The model under review builds one solid part; all positions refer to its coordinate system, in mm. A direction names the side the tool comes from. Give positions to 0.01 mm unless a question says otherwise; leave off trailing zeros. Loops run counter-clockwise (first coordinate to the right, second up) from the corner with the lowest first, then second, coordinate; pieces in that order, holes last. Notation, with made-up numbers: M -22.75,69 L 8.25,69 A20 ccw 8.25,105 Z; hole C 17.5,50.5 d6. An arc over 180 degrees is marked long. Write item = value, one per line. Start each with the question number.
1. We need section C-C on x = 112. Give the boundary of the cut face in (y, z), then the cut area to 3 significant figures.
2. Wall thickness on line 1 along Y through (x, z) = (665.5, 305); line 2 along Z through (x, y) = (-31, 529.5); line 3 along Y through (x, z) = (146, -75): over which ranges is each line inside the solid? List them lowest first. Write a range as from..to.
3. For pin 1 (4 mm diameter, centred on x = -490, y = 935, fed in from +Z); pin 2 (15 mm diameter, centred on y = 1233.5, z = 115.5, fed in from -X); pin 3 (10 mm diameter, centred on x = -468.5, y = 1127, fed in from -Z), all flat-tipped, find the tip position at first contact; note any pin that passes through.
4. For faces 4 (the face through (155, 644, 469.245)), 5 (the face through (-22, 911, 314.233)), 6 (the face through (0, 626, -786)), 7 (the face through (324, 1245, -342.245)), list the 3-axis set-ups (+Z, -Z, +X, -X, +Y, -Y) from which the entire face can be reached by the end or side of a thin tool; tool diameter is ignored.
5. Draft analysis for pull direction Z (two halves, no side actions). For faces 1 (the face through (324, 1219.2, -5)), 2 (the face through (-914.18, 626.11, -20.11)), 3 (the face through (792.47, 503, 7)), state which applies: pulls with the +Z half, pulls with the -Z half, needs draft (parallel to the pull), parting line crosses it, or undercut.
6. We need section B-B on x = -281.5. Count the separate pieces of the cut face and the enclosed holes in it, then the cut area to 3 significant figures.
from build123d import *
from OCP.BRepAlgoAPI import BRepAlgoAPI_Cut
from OCP.TopTools import TopTools_ListOfShape

# Parameters (mm, degrees)
EXTRUDE_1_DEPTH     = 1270
SKETCH_5_W          = 72.235282366
SKETCH_5_H          = 338.817872049
EXTRUDE_1_2_DEPTH   = 1270
SKETCH_9_W          = 66.439449902
SKETCH_9_H          = 119.69450016
EXTRUDE_2_DEPTH     = 1270
SKETCH_779_W        = 1584.940783878
SKETCH_779_H        = 679.265773974
EXTRUDE_7_DEPTH     = 1270.000001702
SKETCH_15_W         = 628.465773974
SKETCH_15_H         = 508
CUT_EXTRUDE_1_DEPTH = 5080
SKETCH_16_W         = 1396.738419433
SKETCH_16_H         = 129.612550511
EXTRUDE_8_DEPTH     = 1270
SKETCH_17_W         = 1408.739581517
SKETCH_17_H         = 129.612550511
EXTRUDE_9_DEPTH     = 1270
SKETCH_20_W         = 622.659597216
SKETCH_20_H         = 684.490874996
CUT_EXTRUDE_2_DEPTH = 50.8


with BuildPart() as part:
    # 草圖1 → Extrude 1 (new body)
    with BuildSketch(Plane(origin=(0, 0, 0), x_dir=(1, 0, 0), z_dir=(0, 1, 0))):
        with BuildLine():
            ThreePointArc((0, 914.4), (-914.4, 0), (0, -914.4))
            Line((0, -914.4), (0, -660.4))
            ThreePointArc((0, -660.4), (-660.4, 0), (0, 660.4))
            Line((0, 660.4), (0, 914.4))
        make_face()
    extrude(amount=EXTRUDE_1_DEPTH)

    # 草圖5 → Extrude 1 2 (add, through all)
    with BuildSketch(Plane(origin=(0, 1270, 0), x_dir=(1, 0, 0), z_dir=(0, 1, 0))):
        with Locations((-828.280286412, 6.324353143)):
            Rectangle(SKETCH_5_W, SKETCH_5_H)
    extrude(amount=-EXTRUDE_1_2_DEPTH)

    # 草圖9 → 填補2 (add, through all)
    with BuildSketch(Plane(origin=(0, 1270, 0), x_dir=(1, 0, 0), z_dir=(0, 1, 0))):
        with Locations((-825.38237018, -198.335355397)):
            Rectangle(SKETCH_9_W, SKETCH_9_H)
    extrude(amount=-EXTRUDE_2_DEPTH)

    # Sketch 779 → 填料-伸長7 (add)
    with BuildSketch(Plane(origin=(0, 0, 0), x_dir=(1, 0, 0), z_dir=(0, 1, 0))):
        Rectangle(SKETCH_779_W, SKETCH_779_H)
    extrude(amount=EXTRUDE_7_DEPTH)

    # 草圖15 → 除料-伸長1 (cut)
    with BuildSketch(Plane(origin=(792.470391939, 0, 0), x_dir=(0, 0, -1), z_dir=(1, 0, 0))):
        with Locations((0, 914.400001702)):
            Rectangle(SKETCH_15_W, SKETCH_15_H)
    extrude(amount=-CUT_EXTRUDE_1_DEPTH, mode=Mode.SUBTRACT)

    # 草圖16 → 填料-伸長8 (add, through all)
    with BuildSketch(Plane(origin=(0, 1270, 0), x_dir=(1, 0, 0), z_dir=(0, 1, 0))):
        with Locations((94.101182222, -404.439162243)):
            Rectangle(SKETCH_16_W, SKETCH_16_H)
    extrude(amount=-EXTRUDE_8_DEPTH)

    # 草圖17 → 填料-伸長9 (add, through all)
    with BuildSketch(Plane(origin=(0, 1270, 0), x_dir=(1, 0, 0), z_dir=(0, 1, 0))):
        with Locations((88.100601181, 404.439162243)):
            Rectangle(SKETCH_17_W, SKETCH_17_H)
    extrude(amount=-EXTRUDE_9_DEPTH)


with BuildPart() as cut_extrude_2_tool:
    # 草圖20 → 除料-伸長2 (new body)
    with BuildSketch(Plane(origin=(0, 1270, 0), x_dir=(1, 0, 0), z_dir=(0, 1, 0))):
        with Locations((328.740593331, 0)):
            Rectangle(SKETCH_20_W, SKETCH_20_H)
    extrude(amount=-CUT_EXTRUDE_2_DEPTH)


with BuildPart() as part_1:
    add(part.part)

    # 除料-伸長2: cut by cut_extrude_2_tool, with a tolerance
    cut_extrude_2_stock = TopTools_ListOfShape()
    cut_extrude_2_stock.Append(part_1.part.wrapped)
    cut_extrude_2_tools = TopTools_ListOfShape()
    cut_extrude_2_tools.Append(cut_extrude_2_tool.part.wrapped)
    cut_extrude_2_cut = BRepAlgoAPI_Cut()
    cut_extrude_2_cut.SetArguments(cut_extrude_2_stock)
    cut_extrude_2_cut.SetTools(cut_extrude_2_tools)
    cut_extrude_2_cut.SetFuzzyValue(0.00001)
    cut_extrude_2_cut.Build()
    add(Compound.cast(cut_extrude_2_cut.Shape()).solids(), mode=Mode.REPLACE)


solid = part_1.part
Final values:
q1.outline = M 0,-469.25 L 1270,-469.25 L 1270,-342.25 L 1219.2,-342.25 L 1219.2,342.25 L 1270,342.25 L 1270,469.25 L 0,469.25 Z; hole M 660.4,-314.23 L 1168.4,-314.23 L 1168.4,314.23 L 660.4,314.23 Z
q1.area = 838,000 mm²
q2.line_1 = 0..660.4, 1168.4..1270
q2.line_2 = -913.87..-659.67, -469.25..469.25, 659.67..913.87
q2.line_3 = 0..660.4, 1168.4..1219.2
q3.pin_1 = 773.29
q3.pin_2 = -908
q3.pin_3 = -788.22
q4.face_4 = +X, +Y, -Y
q4.face_5 = +X, -X
q4.face_6 = -Z, +X, +Y, -Y
q4.face_7 = +Y
q5.face_1 = undercut
q5.face_2 = parting line crosses it
q5.face_3 = needs draft
q6.separate_pieces = 3
q6.enclosed_holes = 1
q6.area = 1,570,000 mm²
